Here's how the part is built. I have some questions about the finished solid (model axes, mm). A direction names the side the tool comes from. Give positions to 0.01 mm unless a question says otherwise; leave off trailing zeros. Write each loop counter-clockwise with the first axis right and the second up, starting at its lowest first coordinate (ties: lowest second). Pieces come first, ordered by that corner, then holes. Notation, with made-up numbers: (-4, 9.5) -> (26, 9.5) arc R17 cw to (26, 36.5) -> close; hole circle Ø5 at (34.5, 34.5). An arc over 180 degrees is marked (long way). Use CSV: the item, a comma, the result in double quotes. Start each with the question number.
(1) Suppose I cut it at D-D on x = 23. List the corners of the cut face in (y, z) for me.
(2) Which directions (+Z, -Z, +X, -X, +Y, -Y) give clear straight access to the entire face, cutting with the end or side of a thin tool? Please do faces 4 (the cylindrical face through (36.212, 8.278, 197.605)), 5 (the flat face through (78, 5, 200)), 6 (the flat face through (79, 10, 0)), 7 (the flat face through (66, 23, 10)).
(3) I need wall thicknesses on L1, parallel to X at y = 37, z = 67.5; L2, parallel to Z at x = 45, y = 30.5; L3, parallel to Z at x = -34.5, y = 22.5. Which ranges of each line are inside material? Lowest first, please. Write a range as [from, to].
(4) Suppose I cut it at B-B on x = -91. List the corners of the cut face in (y, z) for me.
(5) For pin 1 Ø3 at (y, z) = (7, -2) entering from -X; pin 2 Ø1.5 at (x, z) = (76.5, 202.5) entering from -Y; pin 3 Ø3 at (x, y) = (81, 7) entering from +Z; pin 4 Ø5 at (x, y) = (69.41, 22.94) entering from -Z, each with a flat end and sliding along its axis, tell me the tip position at first contact or that it passes through.
(6) Suppose I cut it at A-A on y = 42. List the corners of the cut face in (x, z) for me, plus the area to 3 significant figures.
(7) If we mould it in two halves opening along X, with no side actions, what happens to faces 1 (the cylindrical face through (66.41, 23.07, 98.74)), 2 (the flat face through (79, 5, 5)), 3 (the flat face through (-95.796, 31, 0))? For each: pulls with the +X half, pulls with the -X half, needs draft (parallel to the pull), parting line crosses it, or undercut.
(8) Suppose I cut it at C-C on z = 38. List the corners of the cut face in (x, y) for me, plus the area to 3 significant figures.
from build123d import *

# Parameters (mm, degrees)
ESQUISSE1_R             = 3
BOSS_EXTRU_1_DEPTH      = 200
ESQUISSE4_W             = 5
ESQUISSE4_H             = 50
BOSS_EXTRU_4_DEPTH      = 180
BOSS_EXTRU_7_DEPTH      = 50
ESQUISSE6_W             = 20
ESQUISSE6_H             = 10.719834163
ENL_V_MAT_EXTRU_2_DEPTH = 10
ESQUISSE5_W             = 10
ESQUISSE5_H             = 10
ENL_V_MAT_EXTRU_1_DEPTH = 10
ESQUISSE14_R            = 5
ENL_V_MAT_EXTRU_4_DEPTH = 15
BOSS_EXTRU_8_REACH      = 242.401


with BuildPart() as part:
    # Esquisse1 → Boss.-Extru.1 (new body)
    with BuildSketch(Plane.XY):
        Polygon((-105.796013405, 0), (84.203986595, 0), (84.203986595, 33.502126335), (-105.796013405, 2), align=None)
        with Locations((69.406004871, 22.939397164)):
            Circle(ESQUISSE1_R, mode=Mode.SUBTRACT)
        with Locations((40.981469067, 6.77616521)):
            Circle(ESQUISSE1_R, mode=Mode.SUBTRACT)
        with Locations((-40.796013405, 6)):
            Circle(ESQUISSE1_R, mode=Mode.SUBTRACT)
        with Locations((8.861542866, 12.901085106)):
            Circle(ESQUISSE1_R, mode=Mode.SUBTRACT)
    extrude(amount=BOSS_EXTRU_1_DEPTH)

    # Esquisse4 → Boss.-Extru.4 (add)
    with BuildSketch(Plane(origin=(84.203986595, 0, 0), x_dir=(0, 0, -1), z_dir=(1, 0, 0))):
        with Locations((-202.5, 25)):
            Rectangle(ESQUISSE4_W, ESQUISSE4_H)
        with Locations((2.5, 25)):
            Rectangle(ESQUISSE4_W, ESQUISSE4_H)
    extrude(amount=-BOSS_EXTRU_4_DEPTH)

    # Esquisse8 → Boss.-Extru.7 (add)
    with BuildSketch(Plane(origin=(0, 50, 0), x_dir=(1, 0, 0), z_dir=(0, 1, 0))):
        Polygon((84.203986595, 0), (-95.796013405, 0), (-95.796013405, -5), align=None)
    boss_extru_7 = extrude(amount=-BOSS_EXTRU_7_DEPTH)

    # Esquisse6 → Enlèv. mat.-Extru.2 (cut)
    with BuildSketch(Plane(origin=(0, 0, -5), x_dir=(-1, 0, 0), z_dir=(0, 0, -1))):
        with Locations((95.796013405, 5.359917081)):
            Rectangle(ESQUISSE6_W, ESQUISSE6_H)
    enl_v_mat_extru_2 = extrude(amount=-ENL_V_MAT_EXTRU_2_DEPTH, mode=Mode.SUBTRACT)

    # Esquisse5 → Enlèv. mat.-Extru.1 (cut)
    with BuildSketch(Plane(origin=(84.203986595, 0, 0), x_dir=(0, 0, -1), z_dir=(1, 0, 0))):
        with Locations((-200, 5)):
            Rectangle(ESQUISSE5_W, ESQUISSE5_H)
        with Locations((0, 5)):
            Rectangle(ESQUISSE5_W, ESQUISSE5_H)
    extrude(amount=-ENL_V_MAT_EXTRU_1_DEPTH, mode=Mode.SUBTRACT)

    # Esquisse14 → Enlèv. mat.-Extru.4 (cut)
    with BuildSketch(Plane(origin=(0, 0, -5), x_dir=(-1, 0, 0), z_dir=(0, 0, -1))):
        with Locations((-69.406004871, 22.939397164)):
            Circle(ESQUISSE14_R)
        with Locations((-40.981469067, 6.77616521)):
            Circle(ESQUISSE14_R)
        with Locations((-8.861542866, 12.901085106)):
            Circle(ESQUISSE14_R)
        with Locations((40.796013405, 6)):
            Circle(ESQUISSE14_R)
    enl_v_mat_extru_4 = extrude(amount=-ENL_V_MAT_EXTRU_4_DEPTH, mode=Mode.SUBTRACT)

    # Symétrie3: Boss.-Extru.7, Enlèv. mat.-Extru.2, Enlèv. mat.-Extru.4 across plane
    add(boss_extru_7.mirror(Plane(origin=(0, 0, 100), x_dir=(1, 0, 0), z_dir=(0, 0, -1))))
    add(enl_v_mat_extru_2.mirror(Plane(origin=(0, 0, 100), x_dir=(1, 0, 0), z_dir=(0, 0, -1))), mode=Mode.SUBTRACT)
    add(enl_v_mat_extru_4.mirror(Plane(origin=(0, 0, 100), x_dir=(1, 0, 0), z_dir=(0, 0, -1))), mode=Mode.SUBTRACT)

    # Boss.-Extru.8: up to this plane
    boss_extru_8_end = Plane(origin=(-95.796013405, -180.069431054, 195), z_dir=(-0.0277670672403533, 0, 0.9996144206527183))
    # Esquisse15 → Boss.-Extru.8 (add, up to the surface)
    with BuildSketch(Plane(origin=(0, 0, -5), x_dir=(-1, 0, 0), z_dir=(0, 0, -1)), mode=Mode.PRIVATE) as boss_extru_8_sk1:
        Polygon((-84.203986595, 33.502126335), (-79.203986595, 32.67312301), (-79.203986595, 50), (-84.203986595, 50), align=None)
    boss_extru_8_tool1 = split(extrude(boss_extru_8_sk1.sketch, amount=-BOSS_EXTRU_8_REACH, mode=Mode.PRIVATE), bisect_by=boss_extru_8_end, keep=Keep.BOTH, mode=Mode.PRIVATE)
    add(boss_extru_8_tool1.solids().sort_by_distance((81.683563, 41.542119, -5))[0])


solid = part.part
Geometry says:
1,outline,"(0, -5) -> (50, -5) -> (50, 1.7) -> (23.35, 1.7) -> (23.35, 198.3) -> (50, 198.3) -> (50, 205) -> (0, 205) -> close"
2,face 4,"+Z"
2,face 5,"+Z, +X, -Y"
2,face 6,"-Z, +X, -Y"
2,face 7,"-Z"
3,L1,"[79.2, 84.2]"
3,L2,"[-5, 1.09], [198.91, 205]"
3,L3,"[-5, 3.3], [196.7, 205]"
4,outline,"(0, 5) -> (4.45, 5) -> (4.45, 195) -> (0, 195) -> close; (10.72, -5) -> (50, -5) -> (50, 4.87) -> (10.72, 4.87) -> close; (10.72, 195.13) -> (50, 195.13) -> (50, 205) -> (10.72, 205) -> close"
5,pin 1,"x = -85.8"
5,pin 2,"y = 10"
5,pin 3,"z = 200"
5,pin 4,"through"
6,outline,"(-95.8, -5) -> (84.2, -5) -> (84.2, 205) -> (-95.8, 205) -> (-95.8, 195) -> (79.2, 199.86) -> (79.2, 0.14) -> (-95.8, 5) -> close"
6,area,"3,700 mm²"
7,face 1,"undercut"
7,face 2,"needs draft"
7,face 3,"pulls with the -X half"
8,outline,"(-105.8, 0) -> (84.2, 0) -> (84.2, 50) -> (79.2, 50) -> (79.2, 32.67) -> (-105.8, 2) -> close; hole circle Ø6 at (-40.8, 6); hole circle Ø6 at (8.86, 12.9); hole circle Ø6 at (40.98, 6.78); hole circle Ø6 at (69.41, 22.94)"
8,area,"3,340 mm²"
